```python
from build123d import *

# Parameters (mm, degrees)
SCHIZZO1_W                   = 40
SCHIZZO1_H                   = 20
ESTRUSIONE_ESTRUSIONE2_DEPTH = 8
TAGLIO_ESTRUSIONE4_DEPTH     = 6
ESTRUSIONE_ESTRUSIONE4_DEPTH = 2.5
SCHIZZO7_W                   = 39
SCHIZZO7_H                   = 19
ESTRUSIONE_ESTRUSIONE3_DEPTH = 0.5
SCHIZZO8_W                   = 11
SCHIZZO8_H                   = 16
ESTRUSIONE_ESTRUSIONE5_DEPTH = 0.5
SCHIZZO9_R                   = 6.5
ESTRUSIONE_ESTRUSIONE6_DEPTH = 1
SCHIZZO10_R                  = 5.5
ESTRUSIONE_ESTRUSIONE7_DEPTH = 0.5
SCHIZZO11_R                  = 3
TAGLIO_ESTRUSIONE5_DEPTH     = 26.377155081
SCHIZZO12_R                  = 1.5
ESTRUSIONE_ESTRUSIONE8_DEPTH = 2.5
SCHIZZO13_W                  = 7.322091749
SCHIZZO13_H                  = 2
TAGLIO_ESTRUSIONE6_DEPTH     = 31.020826105
SPECCHIA4_COPY_1_SKETCH_W    = 7.322091749
SPECCHIA4_COPY_1_SKETCH_H    = 2
SPECCHIA4_COPY_1_DEPTH       = 31.020826105
NERVATURA1_REACH             = 33.193
SCHIZZO16_WALL_W             = 71.666005732
SCHIZZO16_WALL_H             = 2


with BuildPart() as part:
    # Schizzo1 → Estrusione-Estrusione2 (new body)
    with BuildSketch(Plane(origin=(0, 0, 0), x_dir=(1, 0, 0), z_dir=(0, 1, 0))):
        Rectangle(SCHIZZO1_W, SCHIZZO1_H)
    extrude(amount=ESTRUSIONE_ESTRUSIONE2_DEPTH)

    # Schizzo2 → Taglio-Estrusione4 (cut)
    with BuildSketch(Plane(origin=(0, 0, 0), x_dir=(1, 0, 0), z_dir=(0, 1, 0))):
        Polygon((16, -8), (-16, -8), (-16, -6), (-18, -6), (-18, 6), (-16, 6), (-16, 8), (16, 8), (16, 6), (18, 6), (18, -6), (16, -6), align=None)
    extrude(amount=TAGLIO_ESTRUSIONE4_DEPTH, mode=Mode.SUBTRACT)

    # Schizzo3 → Foro per Vite M1-1 (revolve, cut)
    with BuildSketch(Plane(origin=(-17.375, 0, 7.375), x_dir=(0, 0, -1), z_dir=(1, 0, 0))):
        Polygon((0, 0), (0, 5.390559402), (0.65, 5), (0.65, 0.025), (0.675, 0), align=None)
    foro_per_vite_m1_1 = revolve(axis=Axis((-17.375, -6.35, 7.375), (0, 1, 0)), mode=Mode.SUBTRACT)

    # Specchia1: Foro per Vite M1-1 across plane
    add(foro_per_vite_m1_1.mirror(Plane(origin=(0, 0, 0), x_dir=(0, 0, 1), z_dir=(1, 0, 0))), mode=Mode.SUBTRACT)

    # Specchia2: Foro per Vite M1-1 across plane
    add(foro_per_vite_m1_1.mirror(Plane.XY), mode=Mode.SUBTRACT)

    # Specchia2 copy 1 sketch → Specchia2 copy 1 (revolve, cut)
    with BuildSketch(Plane(origin=(17.375, 0, -7.375), x_dir=(0, 0, 1), z_dir=(-1, 0, 0))):
        Polygon((0, 0), (0, 5.390559402), (0.65, 5), (0.65, 0.025), (0.675, 0), align=None)
    revolve(axis=Axis((17.375, -6.35, -7.375), (0, 1, 0)), mode=Mode.SUBTRACT)

    # Taglia-Sweep3: sweep along a path in Schizzo5
    with BuildLine(Plane.XZ) as taglia_sweep3_path:
        Line((19, -9), (-19, -9))
        Line((-19, -9), (-19, 9))
        Line((-19, 9), (19, 9))
        Line((19, 9), (19, -9))
    # Schizzo4 → Taglia-Sweep3 (sweep, cut)
    with BuildSketch(Plane.XY):
        with BuildLine():
            Line((-19.25, 0), (-18.75, 0))
            ThreePointArc((-18.75, 0), (-19, 0.25), (-19.25, 0))
        make_face()
    sweep(path=taglia_sweep3_path.line, transition=Transition.RIGHT, mode=Mode.SUBTRACT)

    # Schizzo6 → Estrusione-Estrusione4 (add)
    with BuildSketch(Plane(origin=(0, 8, 0), x_dir=(1, 0, 0), z_dir=(0, 1, 0))):
        with BuildLine():
            Line((5.641101056, 9), (-15, 9))
            Line((-15, 9), (-15, 5))
            ThreePointArc((-15, 5), (-17, 0), (-15, -5))
            Line((-15, -5), (-15, -9))
            Line((-15, -9), (5.641101056, -9))
            ThreePointArc((5.641101056, -9), (20, 0), (5.641101056, 9))
        make_face()
    extrude(amount=ESTRUSIONE_ESTRUSIONE4_DEPTH)

    # Schizzo7 → Estrusione-Estrusione3 (add)
    with BuildSketch(Plane(origin=(0, 8, 0), x_dir=(1, 0, 0), z_dir=(0, 1, 0))):
        Rectangle(SCHIZZO7_W, SCHIZZO7_H)
    extrude(amount=ESTRUSIONE_ESTRUSIONE3_DEPTH)

    # Schizzo8 → Estrusione-Estrusione5 (add)
    with BuildSketch(Plane(origin=(0, 10.5, 0), x_dir=(1, 0, 0), z_dir=(0, 1, 0))):
        with BuildLine():
            Line((-15, 9), (-2, 9))
            Line((-2, 9), (-2, 1.957707578))
            ThreePointArc((-2, 1.957707578), (0.409122281, 0), (-2, -1.957707578))
            Line((-2, -1.957707578), (-2, -9))
            Line((-2, -9), (-15, -9))
            Line((-15, -9), (-15, 9))
        make_face()
        with Locations((-8.5, 0)):
            Rectangle(SCHIZZO8_W, SCHIZZO8_H, mode=Mode.SUBTRACT)
    extrude(amount=ESTRUSIONE_ESTRUSIONE5_DEPTH)

    # Schizzo9 → Estrusione-Estrusione6 (add)
    with BuildSketch(Plane(origin=(0, 10.5, 0), x_dir=(1, 0, 0), z_dir=(0, 1, 0))):
        with Locations(Location((10, 0, 0), (0, 0, 270))):
            Circle(SCHIZZO9_R)
    extrude(amount=ESTRUSIONE_ESTRUSIONE6_DEPTH)

    # Schizzo10 → Estrusione-Estrusione7 (add)
    with BuildSketch(Plane(origin=(0, 11.5, 0), x_dir=(1, 0, 0), z_dir=(0, 1, 0))):
        with Locations(Location((10, 0, 0), (0, 0, 270))):
            Circle(SCHIZZO10_R)
    extrude(amount=ESTRUSIONE_ESTRUSIONE7_DEPTH)

    # Schizzo11 → Taglio-Estrusione5 (cut, through all)
    with BuildSketch(Plane(origin=(0, 12, 0), x_dir=(1, 0, 0), z_dir=(0, 1, 0))):
        with Locations(Location((10, 0, 0), (0, 0, 270))):
            Circle(SCHIZZO11_R)
    extrude(amount=-TAGLIO_ESTRUSIONE5_DEPTH, mode=Mode.SUBTRACT)

    # Schizzo12 → Estrusione-Estrusione8 (add)
    with BuildSketch(Plane(origin=(0, 1, 0), x_dir=(-1, 0, 0), z_dir=(0, -1, 0))):
        with BuildLine():
            Line((-25.5, 9.25), (-20, 9.25))
            Line((-20, 9.25), (-20, -9.25))
            Line((-20, -9.25), (-25.5, -9.25))
            ThreePointArc((-25.5, -9.25), (-26.560660172, -8.810660172), (-27, -7.75))
            Line((-27, -7.75), (-27, 7.75))
            ThreePointArc((-27, 7.75), (-26.560660172, 8.810660172), (-25.5, 9.25))
        make_face()
        with Locations(Location((-24.5, 5, 0), (0, 0, 90))):
            Circle(SCHIZZO12_R, mode=Mode.SUBTRACT)
        with Locations(Location((-24.5, -5, 0), (0, 0, 90))):
            Circle(SCHIZZO12_R, mode=Mode.SUBTRACT)
    estrusione_estrusione8 = extrude(amount=-ESTRUSIONE_ESTRUSIONE8_DEPTH)

    # Schizzo13 → Taglio-Estrusione6 (cut, through all)
    with BuildSketch(Plane(origin=(0, 3.5, 0), x_dir=(1, 0, 0), z_dir=(0, 1, 0))):
        with Locations((30.661045875, 5)):
            Rectangle(SCHIZZO13_W, SCHIZZO13_H)
        with BuildLine():
            Line((25.618033989, 4), (27, 4))
            Line((27, 4), (27, 6))
            Line((27, 6), (25.618033989, 6))
            ThreePointArc((25.618033989, 6), (25.645827846, 5.968028175), (25.672707741, 5.93528421))
            ThreePointArc((25.672707741, 5.93528421), (25.915814538, 5.495448478), (26, 5))
            ThreePointArc((26, 5), (25.915814538, 4.504551522), (25.672707741, 4.06471579))
            ThreePointArc((25.672707741, 4.06471579), (25.645827846, 4.031971825), (25.618033989, 4))
        make_face()
    taglio_estrusione6 = extrude(amount=-TAGLIO_ESTRUSIONE6_DEPTH, mode=Mode.SUBTRACT)

    # Specchia3: Taglio-Estrusione6 across plane
    add(taglio_estrusione6.mirror(Plane.XY), mode=Mode.SUBTRACT)

    # Specchia4: Estrusione-Estrusione8, Taglio-Estrusione6 across plane
    add(estrusione_estrusione8.mirror(Plane(origin=(0, 0, 0), x_dir=(0, 0, 1), z_dir=(1, 0, 0))))
    add(taglio_estrusione6.mirror(Plane(origin=(0, 0, 0), x_dir=(0, 0, 1), z_dir=(1, 0, 0))), mode=Mode.SUBTRACT)

    # Specchia4 copy 1 sketch → Specchia4 copy 1 (cut, through all)
    with BuildSketch(Plane(origin=(0, 3.5, 0), x_dir=(-1, 0, 0), z_dir=(0, 1, 0))):
        with Locations((30.661045875, 5)):
            Rectangle(SPECCHIA4_COPY_1_SKETCH_W, SPECCHIA4_COPY_1_SKETCH_H)
        with BuildLine():
            Line((25.618033989, 4), (27, 4))
            Line((27, 4), (27, 6))
            Line((27, 6), (25.618033989, 6))
            ThreePointArc((25.618033989, 6), (25.645827846, 5.968028175), (25.672707741, 5.93528421))
            ThreePointArc((25.672707741, 5.93528421), (25.915814538, 5.495448478), (26, 5))
            ThreePointArc((26, 5), (25.915814538, 4.504551522), (25.672707741, 4.06471579))
            ThreePointArc((25.672707741, 4.06471579), (25.645827846, 4.031971825), (25.618033989, 4))
        make_face()
    extrude(amount=-SPECCHIA4_COPY_1_DEPTH, mode=Mode.SUBTRACT)

    # Schizzo16 wall → Nervatura1 (add, up to next)
    with BuildSketch(Plane(origin=(23.5, 4.5, 0), x_dir=(-0.961523947641, 0.274721127897, 0), z_dir=(-0.274721127897, -0.961523947641, 0)), mode=Mode.PRIVATE) as nervatura1_sk1:
        Rectangle(SCHIZZO16_WALL_W, SCHIZZO16_WALL_H)
    nervatura1_tool1 = extrude(nervatura1_sk1.sketch, amount=NERVATURA1_REACH, mode=Mode.PRIVATE) - part.part
    nervatura1 = nervatura1_tool1.solids().sort_by_distance((23.5, 4.5, 0))[0]
    add(nervatura1)

    # Specchia5: Nervatura1 across plane
    add(nervatura1.mirror(Plane(origin=(0, 0, 0), x_dir=(0, 0, 1), z_dir=(1, 0, 0))))


solid = part.part
```
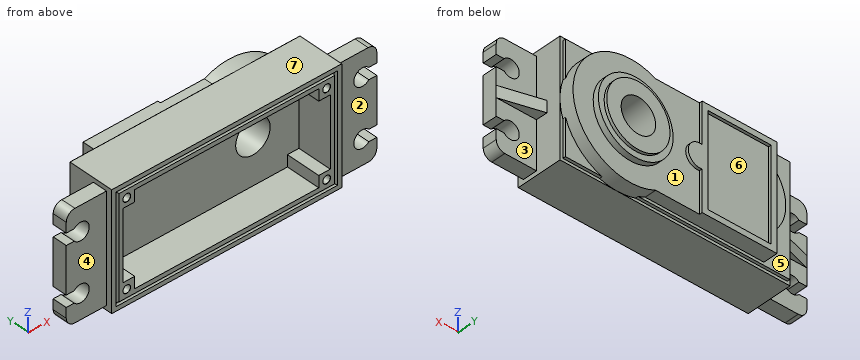
Work out the finished part from the listing and answer in its coordinate system (mm). Face numbers are marked on the shaded views. A direction names the side the tool comes from. Round coordinates to 2 decimals unless told otherwise and drop trailing zeros. Loops run counter-clockwise (first coordinate to the right, second up) from the corner with the lowest first, then second, coordinate; pieces in that order, holes last.
(1) Each of these flat-tipped pins is pushed along its axis until it touches: P1, Ø2, axis at x = -17.375, z = 7.375, coming from the +Y side; P2, Ø3.5, axis at x = 24.5, z = 5, coming from the +Y side; P3, Ø0.6, axis at y = 11, z = 5, coming from the +X side. Where does it stop, or does it pass through?
Computed values:
P1: stops at y = 8.5
P2: stops at y = 3.5
P3: stops at x = 14.49
(2) For the marked faces 1, 2, 3 and 4, determine the directions among +Z, -Z, +X, -X, +Y, -Y from which every point of the face is accessible in a straight line to the end or side of a thin tool.
Computed values:
face 1: +Y
face 2: +Z, -Z, +X, -Y
face 3: -Z, +X, +Y
face 4: +Z, -Z, -X, -Y
(3) Find the intervals of material crossed by L1, parallel to Z at x = 24.5, y = 2.45; L2, parallel to X at y = 5.5, z = -2; L3, parallel to Y at x = 13, z = 5, in increasing order.
Computed values:
L1: z = -9.25 to -6.5, -3.5 to 3.5, 6.5 to 9.25
L2: x = -20 to -18, 18 to 20
L3: y = 6 to 11.5
(4) The part is cut by section C-C, the plane y = 4.5. Give the vertices of the cut face in (x, z) (3 decimals), and give its area (3 significant figures).
Computed values:
outline: (-23.5, -1) - (-20, -1) - (-20, -10) - (20, -10) - (20, -1) - (23.5, -1) - (23.5, 1) - (20, 1) - (20, 10) - (-20, 10) - (-20, 1) - (-23.5, 1) - close; hole circle Ø1.3 at (-17.375, -7.375); hole circle Ø1.3 at (-17.375, 7.375); hole (-18, -6) - (-16, -6) - (-16, -8) - (16, -8) - (16, -6) - (18, -6) - (18, 6) - (16, 6) - (16, 8) - (-16, 8) - (-16, 6) - (-18, 6) - close; hole circle Ø1.3 at (17.375, -7.375); hole circle Ø1.3 at (17.375, 7.375)
area: 249 mm2
(5) The part is cut by section B-B, the plane x = -24.5. Give the vertices of the cut face in (y, z).
Computed values:
outline: (1, -9.25) - (3.5, -9.25) - (3.5, -6.5) - (1, -6.5) - close; (1, -3.5) - (3.5, -3.5) - (3.5, -1) - (4.21, -1) - (4.21, 1) - (3.5, 1) - (3.5, 3.5) - (1, 3.5) - close; (1, 6.5) - (3.5, 6.5) - (3.5, 9.25) - (1, 9.25) - close
(6) The part is cut by section D-D, the plane x = 22.5. Give the vertices of the cut face in (y, z).
Computed values:
outline: (1, -9.25) - (3.5, -9.25) - (3.5, -1) - (4.79, -1) - (4.79, 1) - (3.5, 1) - (3.5, 9.25) - (1, 9.25) - close
(7) The part is cut by section A-A, the plane y = 9.75. Give the vertices of the cut face in (x, z), and give its area (3 significant figures).
Computed values:
outline: (-15, -9) - (5.64, -9) arc R10 ccw (long way) to (5.64, 9) - (-15, 9) - (-15, 5) arc R7.25 ccw to (-15, -5) - close; hole circle Ø6 at (10, 0)
area: 598 mm2
(8) The mould has two halves that part along Z. Classify the marked faces 5, 6 and 7: pulls with the +Z half, pulls with the -Z half, needs draft (parallel to the pull), parting line crosses it, or undercut.
Computed values:
face 5: needs draft
face 6: undercut
face 7: pulls with the +Z half
